Build history of the part. All positions in model axes, mm. A direction names the side the tool comes from. Give positions to 0.01 mm unless a question says otherwise; leave off trailing zeros. Order: outer loops, then holes, each group sorted by start corner. A loop starts at its lowest first (then second) coordinate and runs counter-clockwise, first axis right, second up. Notation, with made-up numbers: M 60.5,-10 L 87.5,-10 A20 ccw 87.5,16 Z; hole C 44,79.25 d4. An arc over 180 degrees is marked long. Answer as CSV lines item,"result".
Autodesk Inventor part; units mm, degrees
ref_plane "YZ Plane" through (0, 0, 0) normal (1, 0, 0) x (0, 1, 0)
ref_plane "XZ Plane" through (0, 0, 0) normal (0, 1, 0) x (-1, 0, 0)
ref_plane "XY Plane" through (0, 0, 0) normal (0, 0, 1) x (1, 0, 0)
sketch "Boceto1" plane through (0, 0, 0) normal (0, 1, 0) x (-1, 0, 0)
  line L0 (0, 5) -> (4.3301, 2.5)
  line L1 (4.3301, 2.5) -> (4.3301, -2.5)
  line L2 (4.3301, -2.5) -> (0, -5)
  line L3 (0, -5) -> (-4.3301, -2.5)
  line L4 (-4.3301, -2.5) -> (-4.3301, 2.5)
  line L5 (-4.3301, 2.5) -> (0, 5)
  circle A0 centre (0, 0) radius 4
  circle A1 centre (0, 0) radius 2
  dimension "d0" = 10
  dimension "d1" = 8
  dimension "d2" = 4
extrude "Extrusión1" add sketch "Boceto1" along normal blind 10 contours L0 L1 L2 L3 L4 L5
extrude "Extrusión2" add sketch "Boceto1" along normal blind 2 contours A0
thread "Rosca1"
properties part number "Pieza 1 subensamble 1-69" material "Latón, amarillo claro"
Item 1: Band-saw the part on A-A (z = 0). Give the cut face in (x, y), and give its area (3 significant figures).
Geometry says:
outline,"M -4.33,0 L -2,0 L -2,2 L -4,2 L -4,10 L -4.33,10 Z; M 2,0 L 4.33,0 L 4.33,10 L 4,10 L 4,2 L 2,2 Z"
area,"14.6 mm2"
Item 2: Pull direction X, two halves, no side cores. Call faces 3 (the flat face through (0.1, 0, -2.2)), 4 (the cylindrical face through (0.867, 5.944, 3.905)), 5 (the flat face through (2.2, 4.93, 3.73)): released by +X, released by -X, zero draft, split by the parting line, or undercut.
Geometry says:
face 3,"zero draft"
face 4,"undercut"
face 5,"released by +X"
Item 3: 3-axis set-ups, long thin cutter, end or side, ignore diameter. For faces 1 (the flat face through (2, 2, -1)), 2 (the cylindrical face through (0, 1, 2)): which of +Z, -Z, +X, -X, +Y, -Y reach the whole face in a straight line?
Geometry says:
face 1,"+Y"
face 2,"+Y, -Y"
Item 4: Probe line 1 along Y through (x, z) = (-1, 3.5); line 2 along Z through (x, y) = (2.75, 3); line 3 along Z through (x, y) = (3, 6.5). List the from-to ranges inside material, lowest first. Write a range as from..to.
Geometry says:
line 1,"y = 0..2"
line 2,"z = -3.41..-2.9, 2.9..3.41"
line 3,"z = -3.27..-2.65, 2.65..3.27"
Item 5: Band-saw the part on D-D (x = -3.25). Give the cut face in (y, z), and give its area (3 significant figures).
Geometry says:
outline,"M 0,-3.12 L 10,-3.12 L 10,-2.33 L 2,-2.33 L 2,2.33 L 10,2.33 L 10,3.12 L 0,3.12 Z"
area,"25.2 mm2"
Item 6: Drop flat-ended pins along their axis: pin 1 (1.5 mm diameter, centred on x = -3, y = 7.5, fed in from +Z); pin 2 (1 mm diameter, centred on x = -2.5, z = -0.5, fed in from +Y). Give the stop position or say it passes through.
Geometry says:
pin 1,"stops at z = 3.7"
pin 2,"stops at y = 2"
Item 7: Band-saw the part on C-C (x = -0.25). Give the cut face in (y, z).
Geometry says:
outline,"M 0,-4.86 L 10,-4.86 L 10,-3.99 L 2,-3.99 L 2,-1.98 L 0,-1.98 Z; M 0,1.98 L 2,1.98 L 2,3.99 L 10,3.99 L 10,4.86 L 0,4.86 Z"
Item 8: Band-saw the part on B-B (y = 4.5). Give the cut face in (x, z), and give its area (3 significant figures).
Geometry says:
outline,"M -4.33,-2.5 L 0,-5 L 4.33,-2.5 L 4.33,2.5 L 0,5 L -4.33,2.5 Z; hole C 0,0 d8"
area,"14.7 mm2"
